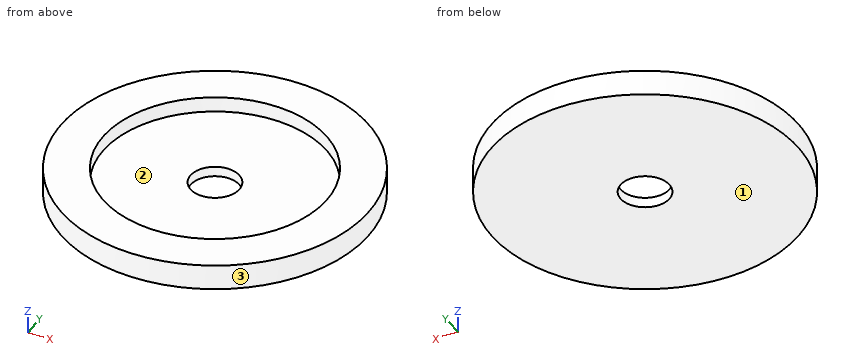
Autodesk Inventor part; units mm, degrees
ref_plane "YZ Plane" through (0, 0, 0) normal (1, 0, 0) x (0, 1, 0)
ref_plane "XZ Plane" through (0, 0, 0) normal (0, 1, 0) x (-1, 0, 0)
ref_plane "XY Plane" through (0, 0, 0) normal (0, 0, 1) x (1, 0, 0)
sketch "Sketch1" plane through (0, 0, 0) normal (0, 0, 1) x (1, 0, 0)
  circle A0 centre (-29.7426, 29.7426) radius 3.2004
  circle A1 centre (29.7426, -29.7426) radius 3.2004
  circle A2 centre (0, 0) radius 8.001
  circle A3 centre (0, 0) radius 50.1904
extrude "Extrusion1" add sketch "Sketch1" along normal blind 8.3312 contours A0 | A1 | A2 | A3
sketch "Sketch2" plane through (0, 0, 8.3312) normal (0, 0, 1) x (1, 0, 0)
  circle A0 centre (0, 0) radius 50.1904
  circle A1 centre (0, 0) radius 36.4998
  dimension "d2" = 72.9996
extrude "Extrusion2" cut sketch "Sketch2" against normal blind 5.0038 contours A1
sketch "Sketch3" plane through (0, 0, 3.3274) normal (0, 0, 1) x (1, 0, 0)
  circle A0 centre (0, 0) radius 36.4998
  circle A1 centre (0, 0) radius 8.001
  dimension "d5" = 16.002
extrude "Extrusion3" cut sketch "Sketch3" against normal through all contours A1
properties part number "top plate washer"
Here's how the part is built. I have some questions about the finished solid (model axes, mm). Face numbers are marked on the shaded views. Coordinates: 2 decimals unless noted, no trailing zeros. Order: outer loops, then holes, each group sorted by start corner. A loop starts at its lowest first (then second) coordinate and runs counter-clockwise, first axis right, second up.
Item 1: If we section it at D-D on y = 29: List the corners of the cut face in (x, z) for me.
Result sheet:
outline: (-40.96, 0) - (40.96, 0) - (40.96, 8.33) - (22.16, 8.33) - (22.16, 3.33) - (-22.16, 3.33) - (-22.16, 8.33) - (-40.96, 8.33) - close
Item 2: If we section it at C-C on z = 5.5: List the corners of the cut face in (x, y) for me.
Result sheet:
outline: circle Ø100.38 at (0, 0); hole circle Ø73 at (0, 0)
Item 3: If we mould it in two halves opening along Y, with no side actions, what happens to the marked faces 1, 2 and 3? For each: +Y half, -Y half, draft (parallel to the pull), parting line (faces both ways), or undercut.
Result sheet:
face 1: draft
face 2: undercut
face 3: parting line
Item 4: I need wall thicknesses on line 1 (Y direction, x = 0, z = 2.6); line 2 (Y direction, x = 0, z = 5.5); line 3 (Z direction, x = -6.5, y = 22). Which ranges of each line are inside material? Lowest first, please.
Result sheet:
line 1: y = -50.19 to -8, 8 to 50.19
line 2: y = -50.19 to -36.5, 36.5 to 50.19
line 3: z = 0 to 3.33
Item 5: If we section it at A-A on x = 0: List the corners of the cut face in (y, z) for me, plus the area to 3 significant figures.
Result sheet:
outline: (-50.19, 0) - (-8, 0) - (-8, 3.33) - (-36.5, 3.33) - (-36.5, 8.33) - (-50.19, 8.33) - close; (8, 0) - (50.19, 0) - (50.19, 8.33) - (36.5, 8.33) - (36.5, 3.33) - (8, 3.33) - close
area: 418 mm2
Item 6: For P1, Ø2, axis at x = -5, z = 4, coming from the +Y side; P2, Ø2, axis at x = -20, z = 6.5, coming from the +Y side; P3, Ø13, axis at x = 0, y = 0, coming from the -Z side; P4, Ø2, axis at x = -6, y = 16.5, coming from the +Z side, each with a flat end and sliding along its axis, tell me the tip position at first contact or that it passes through.
Result sheet:
P1: stops at y = 50.03
P2: stops at y = 46.46
P3: passes through
P4: stops at z = 3.33
